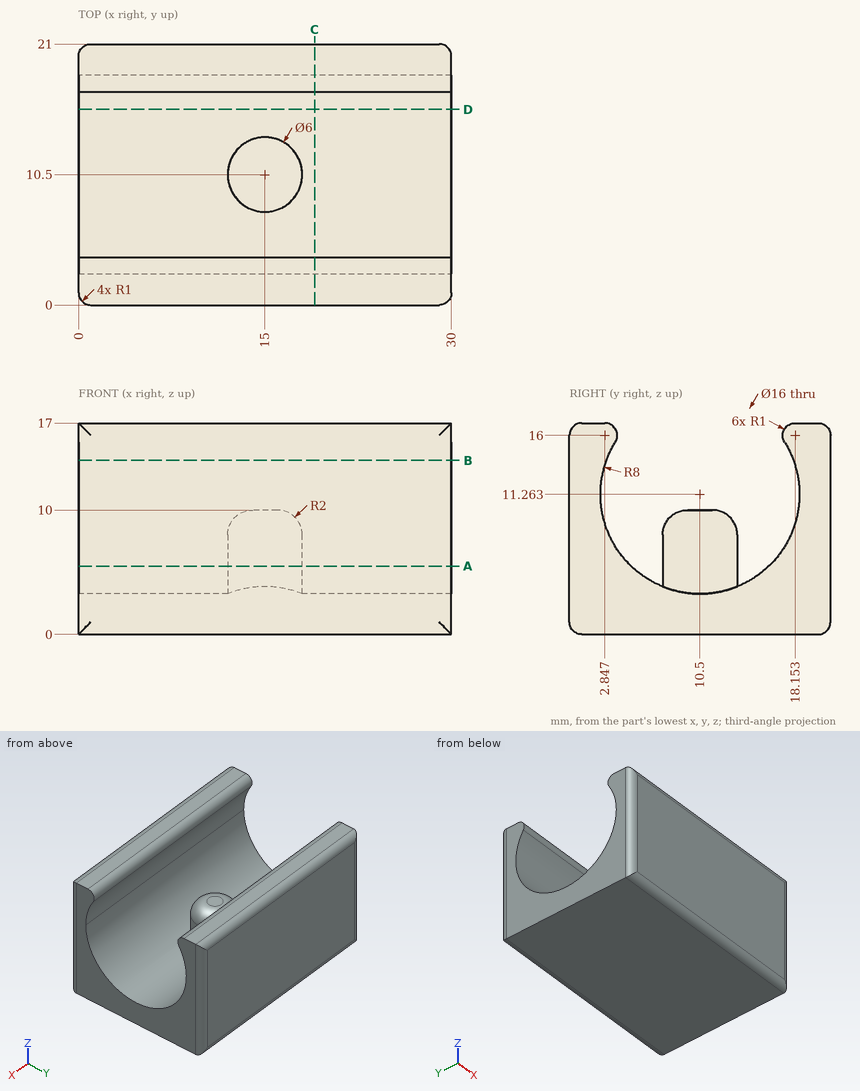
Study the drawing (mm; zero at the part's minimum x, y, z) and answer. Give positions to 0.01 mm unless a question says otherwise; leave off trailing zeros. Write each loop counter-clockwise with the first axis right and the second up, starting at its lowest first coordinate (ties: lowest second). Pieces come first, ordered by that corner, then holes.
Item 1: Find the intervals of material crossed by line 1 along Y through (x, z) = (28.5, 13.75) (1 decimal); line 2 along X through (y, z) = (10.5, 6.75); line 3 along Y through (x, z) = (9, 15.75) (1 decimal), in increasing order.
Item 2: Flat-ended cylindrical pins translate along their axes: P1, Ø1.6, axis at x = 15, y = 10, coming from the +Z side; P2, Ø10, axis at y = 16.5, z = 13.5, coming from the -X side; P3, Ø6, axis at x = 21, y = 12.5, coming from the +Z side; P4, Ø1.5, axis at x = 21.5, y = 16, coming from the +Z side. Find the tip coordinate at first contact, or state that the pin passes through.
Item 3: Section C-C, the plane x = 19 is taken. Write down the section's boundary in (y, z).
Item 4: Section D-D, the plane y = 15.75 is taken. Write down the section's boundary in (x, z), plus the area to 3 significant figures.
Item 5: Section A-A, the plane z = 5.5 is taken. Write down the section's boundary in (x, y).
Item 6: Section B-B, the plane z = 14 is taken. Write down the section's boundary in (x, y), plus the area to 3 significant figures.
Completed:
1. line 1: y = 0 to 2.9, 18.1 to 21
1. line 2: x = 12 to 18
1. line 3: y = 0 to 3.8, 17.2 to 21
2. P1: stops at z = 10
2. P2: stops at x = 0
2. P3: stops at z = 5.02
2. P4: stops at z = 6.27
3. outline: (0, 1) arc R1 ccw to (1, 0) - (20, 0) arc R1 ccw to (21, 1) - (21, 16) arc R1 ccw to (20, 17) - (18.15, 17) arc R1 ccw to (17.3, 15.47) arc R8 cw (long way) to (3.7, 15.47) arc R1 ccw to (2.85, 17) - (1, 17) arc R1 ccw to (0, 16) - close
4. outline: (0, 0) - (30, 0) - (30, 5.23) - (0, 5.23) - close
4. area: 157 mm2
5. outline: (0, 1) arc R1 ccw to (1, 0) - (29, 0) arc R1 ccw to (30, 1) - (30, 4.95) - (0, 4.95) - close; (0, 16.05) - (30, 16.05) - (30, 20) arc R1 ccw to (29, 21) - (1, 21) arc R1 ccw to (0, 20) - close; circle Ø6 at (15, 10.5)
6. outline: (0, 1) arc R1 ccw to (1, 0) - (29, 0) arc R1 ccw to (30, 1) - (30, 2.98) - (0, 2.98) - close; (0, 18.02) - (30, 18.02) - (30, 20) arc R1 ccw to (29, 21) - (1, 21) arc R1 ccw to (0, 20) - close
6. area: 178 mm2
